Design review of the part built by this model. Coordinates are the model's own, in mm. Face numbers are marked on the shaded views. A direction names the side the tool comes from. Give positions to 0.01 mm unless a question says otherwise; leave off trailing zeros. Order: outer loops, then holes, each group sorted by start corner. A loop starts at its lowest first (then second) coordinate and runs counter-clockwise, first axis right, second up. Notation, with made-up numbers: (-17, -16) -> (-8, -16) arc R20 cw to (-8, 15) -> close; hole circle Ø11 at (-31, 11). An arc over 180 degrees is marked (long way). Return JSON: item names as keys, results as strings.
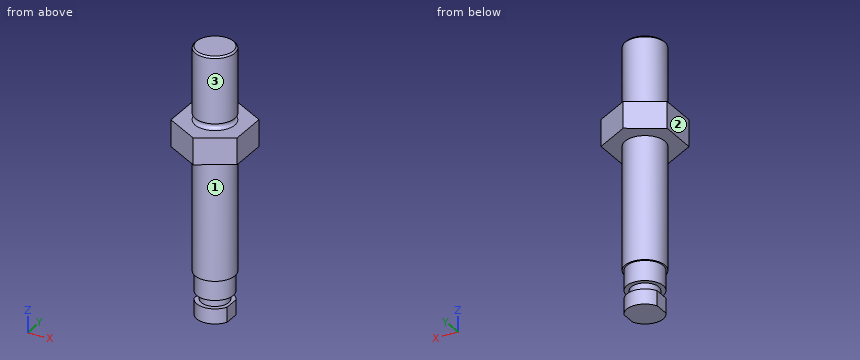
Autodesk Inventor part; units mm, degrees
ref_plane "工作平面1" through (0, 0, -43) normal (0, 0, -1) x (-1, 0, 0)
ref_plane "工作平面6" through (0, 0, 0) normal (0, 1, 0) x (-1, 0, 0)
ref_plane "工作平面8" through (0, 0, 0) normal (1, 0, 0) x (0, 1, 0)
sketch "草圖1" plane through (0, 0, 0) normal (0, 0, 1) x (1, 0, 0)
  line L0 (0, -11.547) -> (-10, -5.7735)
  line L1 (-10, -5.7735) -> (-10, 5.7735)
  line L2 (-10, 5.7735) -> (0, 11.547)
  line L3 (0, 11.547) -> (10, 5.7735)
  line L4 (10, 5.7735) -> (10, -5.7735)
  line L5 (10, -5.7735) -> (0, -11.547)
  point P0 (0, 0)
  point P1 (0, 0)
  dimension "d16" = 20
extrude "擠出1" add sketch "草圖1" along normal blind 8
sketch "草圖2" plane through (0, 0, 8) normal (0, 0, 1) x (1, 0, 0)
  circle A0 centre (0, 0) radius 6
  dimension "d3" = 12
extrude "擠出2" add sketch "草圖2" along normal blind 22
thread "螺紋1"
sketch "草圖3" plane through (0, 0, 0) normal (0, 0, -1) x (-1, 0, 0)
  circle A0 centre (0, 0) radius 6
  dimension "d8" = 12
extrude "擠出3" add sketch "草圖3" along normal blind 50
ref_plane "工作平面1" through (0, 0, -43) normal (0, 0, -1) x (-1, 0, 0)
sketch "草圖4" plane through (0, 0, -43) normal (0, 0, -1) x (-1, 0, 0)
  circle A0 centre (0, 0) radius 4.15
  circle A1 centre (0, 0) radius 6
  dimension "d12" = 8.3
  dimension "d13" = 12
extrude "擠出4" cut sketch "草圖4" along normal blind 2.5
ref_plane "工作平面6" through (0, 0, 0) normal (0, 1, 0) x (-1, 0, 0)
chamfer "倒角1" distance 0.5 angle 45 1 edges at (-6, 0, 30)
ref_plane "工作平面8" through (0, 0, 0) normal (1, 0, 0) x (0, 1, 0)
sketch "草圖7" plane through (0, 0, 0) normal (1, 0, 0) x (0, 1, 0)
  line L0 (-5.5, 30) -> (5.5, 30)
  line L1 (-6, 8) -> (6, 8)
  line L2 (6, 29.5) -> (-6, 29.5)
  line L3 (-6, 8) -> (-6, 9)
  arc A0 (-6, 8) -> (-6, 10) centre (-6, 9) ccw
  line L4 (-6, 10) -> (-6, 8)
  line L5 (0, -6) -> (0, 36)
  point P0 (0, 0)
revolve "迴轉1" cut sketch "草圖7" angle 360 about axis through (0, 0, -10) along (0, 0, 1)
sketch "草圖10" plane through (0, 0, -50) normal (0, 0, -1) x (-1, 0, 0)
  line L0 (-5, -2.2913) -> (-5, 2.2913)
  line L1 (5, 2.2913) -> (5, -2.2913)
  circle A0 centre (0, 0) radius 5.5
  point P0 (5, -2.8868)
  point P1 (-5, -2.8868)
  point P2 (5, 2.8868)
  dimension "d40" = 10
sketch "草圖11" plane through (0, 0, -50) normal (0, 0, -1) x (-1, 0, 0)
  arc A0 (6, 0) -> (6, 0) centre (0, 0) ccw
  circle A1 centre (0, 0) radius 5.5
  circle A2 centre (0, 0) radius 6
  dimension "d45" = 11
extrude "擠出10" cut sketch "草圖11" against normal blind 13
extrude "擠出11" cut sketch "草圖10" against normal up to next contours A0 L0 | L1 A0
properties part number "移動輪固定軸"
Item 1: Add section B-B (z = -42). Give the boundary of the cut face in (x, y).
Result set:
{"outline": "circle Ø11 at (0, 0)"}
Item 2: Machinability: for the marked faces 1, 2 and 3, which of the approach directions +Z, -Z, +X, -X, +Y, -Y give a long, thin tool a straight path to every point of the face, cutting with its end or side? Answer none if there is none.
Result set:
{"face 1": "-Z", "face 2": "+Z, -Z, -X, +Y, -Y", "face 3": "+Z"}
Item 3: Wall thickness on L1, parallel to Z at x = -4.5, y = -4.25; L2, parallel to Y at x = -3.75, z = 26; L3, parallel to Y at x = -0.25, z = 23: over which ranges is each line inside the solid? List them lowest first. Write a range as [from, to].
Result set:
{"L1": "z = [0, 8]", "L2": "y = [-4.68, 4.68]", "L3": "y = [-5.99, 5.99]"}
Item 4: Add section C-C (x = 7). Give the boundary of the cut face in (y, z).
Result set:
{"outline": "(-7.51, 0) -> (7.51, 0) -> (7.51, 8) -> (-7.51, 8) -> close"}
Item 5: Add section A-A (y = 0). Give the boundary of the cut face in (x, z), plus the area to 3 significant figures.
Result set:
{"outline": "(-10, 0) -> (-6, 0) -> (-6, -37) -> (-5.5, -37) -> (-5.5, -43) -> (-4.15, -43) -> (-4.15, -45.5) -> (-5, -45.5) -> (-5, -50) -> (5, -50) -> (5, -45.5) -> (4.15, -45.5) -> (4.15, -43) -> (5.5, -43) -> (5.5, -37) -> (6, -37) -> (6, 0) -> (10, 0) -> (10, 8) -> (6, 8) arc R1 cw to (6, 10) -> (6, 29.5) -> (5.5, 30) -> (-5.5, 30) -> (-6, 29.5) -> (-6, 10) arc R1 cw to (-6, 8) -> (-10, 8) -> close", "area": "996 mm^2"}
Item 6: For pin 1 (4 mm diameter, centred on x = -4.5, z = 21, fed in from +Y); pin 2 (1.5 mm diameter, centred on x = 4, z = -34.5, fed in from +Y); pin 3 (3 mm diameter, centred on x = -2.5, z = -34, fed in from +Y), all flat-tipped, find the tip position at first contact; note any pin that passes through.
Result set:
{"pin 1": "stops at y = 5.45", "pin 2": "stops at y = 5.04", "pin 3": "stops at y = 5.92"}
Item 7: Add section D-D (z = -7). Give the boundary of the cut face in (x, y).
Result set:
{"outline": "circle Ø12 at (0, 0)"}
